CAD build for the part. Positions are in the model's coordinates, mm. A direction names the side the tool comes from. Round coordinates to 2 decimals unless told otherwise and drop trailing zeros. Loops run counter-clockwise (first coordinate to the right, second up) from the corner with the lowest first, then second, coordinate; pieces in that order, holes last.
Autodesk Inventor part; units mm, degrees
ref_plane "YZ Plane" through (0, 0, 0) normal (1, 0, 0) x (0, 1, 0)
ref_plane "XZ Plane" through (0, 0, 0) normal (0, 1, 0) x (-1, 0, 0)
ref_plane "XY Plane" through (0, 0, 0) normal (0, 0, 1) x (1, 0, 0)
sketch "Sketch1" plane through (0, 0, 0) normal (0, 0, 1) x (1, 0, 0)
  line L0 (-300, 0) -> (300, 0)
  line L1 (300, 0) -> (300, 1900)
  line L2 (300, 1900) -> (-300, 1900)
  line L3 (-300, 1900) -> (-300, 0)
  point P0 (0, 0)
  point P1 (0, 0)
  dimension "d0" = 600
  dimension "d1" = 1900
extrude "Extrusion1" add sketch "Sketch1" along normal blind 330
sketch "Sketch2" plane through (-300, 1900, 0) normal (0, 1, 0) x (1, 0, 0)
  line L0 (600, 0) -> (0, 0) construction
  line L1 (0, 0) -> (0, -330) construction
  line L2 (600, -330) -> (0, -330) construction
  line L3 (600, 0) -> (600, -330) construction
  line L4 (0, 0) -> (600, 0)
  line L5 (600, 0) -> (600, -350)
  line L6 (600, -350) -> (0, -350)
  line L7 (0, -350) -> (0, 0)
  point P0 (300, 0)
  dimension "d4" = 350
extrude "Extrusion2" add sketch "Sketch2" against normal blind 17.5
sketch "Sketch3" plane through (0, 0, 330) normal (0, 0, 1) x (1, 0, 0)
  line L0 (300, 1882.5) -> (-300, 1882.5)
  line L1 (-282.5, 1882.5) -> (282.5, 1882.5)
  line L2 (282.5, 1882.5) -> (282.5, 1575)
  line L3 (282.5, 1575) -> (-282.5, 1575)
  line L4 (-282.5, 1575) -> (-282.5, 1882.5)
  line L5 (-282.5, 1557.5) -> (282.5, 1557.5)
  line L6 (282.5, 1557.5) -> (282.5, 1250)
  line L7 (282.5, 1250) -> (-282.5, 1250)
  line L8 (-282.5, 1250) -> (-282.5, 1557.5)
  line L9 (282.5, 1232.5) -> (-282.5, 1232.5)
  line L10 (-282.5, 1232.5) -> (-282.5, 925)
  line L11 (-282.5, 925) -> (282.5, 925)
  line L12 (282.5, 925) -> (282.5, 1232.5)
  line L13 (-282.5, 907.5) -> (282.5, 907.5)
  line L14 (282.5, 907.5) -> (282.5, 600)
  line L15 (282.5, 600) -> (-282.5, 600)
  line L16 (-282.5, 600) -> (-282.5, 907.5)
  line L17 (-300, 0) -> (300, 0)
  line L18 (-282.5, 1575) -> (-282.5, 1557.5) construction
  line L19 (-282.5, 1250) -> (-282.5, 1232.5) construction
  line L20 (-282.5, 925) -> (-282.5, 907.5) construction
  point P0 (0, 0)
  point P1 (0, 600)
  point P2 (0, 0)
  dimension "d7" = 600
  dimension "d8" = 17.5
  dimension "d9" = 565
extrude "Extrusion3" cut sketch "Sketch3" against normal blind 312.5
properties part number "Libreria"
Item 1: Cut at A-A (x = 215). List the corners of the cut face in (y, z).
Verdict:
outline: (0, 0) - (1900, 0) - (1900, 350) - (1882.5, 350) - (1882.5, 17.5) - (1575, 17.5) - (1575, 330) - (1557.5, 330) - (1557.5, 17.5) - (1250, 17.5) - (1250, 330) - (1232.5, 330) - (1232.5, 17.5) - (925, 17.5) - (925, 330) - (907.5, 330) - (907.5, 17.5) - (600, 17.5) - (600, 330) - (0, 330) - close
Item 2: Wall check: L1, parallel to Y at x = -109.5, z = 62; L2, parallel to X at y = 1537, z = 296; L3, parallel to Z at x = 119.5, y = 1689. Give the ranges that are in metal, low to high.
Verdict:
L1: y = 0 to 600, 907.5 to 925, 1232.5 to 1250, 1557.5 to 1575, 1882.5 to 1900
L2: x = -300 to -282.5, 282.5 to 300
L3: z = 0 to 17.5
Item 3: Cut at C-C (y = 1175.5). List the corners of the cut face in (x, z).
Verdict:
outline: (-300, 0) - (300, 0) - (300, 330) - (282.5, 330) - (282.5, 17.5) - (-282.5, 17.5) - (-282.5, 330) - (-300, 330) - close
Item 4: Cut at D-D (y = 530). List the corners of the cut face in (x, z), plus the area to 3 significant figures.
Verdict:
outline: (-300, 0) - (300, 0) - (300, 330) - (-300, 330) - close
area: 198,000 mm2
Item 5: Flat gauge pin, fed straight in: P1, Ø3, axis at x = 230.5, y = 1240.5, coming from the +Z side. Where does the tip first touch, or does it go through?
Verdict:
P1: stops at z = 330
Item 6: Cut at B-B (z = 230). List the corners of the cut face in (x, y).
Verdict:
outline: (-300, 0) - (300, 0) - (300, 1900) - (-300, 1900) - close; hole (-282.5, 600) - (282.5, 600) - (282.5, 907.5) - (-282.5, 907.5) - close; hole (-282.5, 925) - (282.5, 925) - (282.5, 1232.5) - (-282.5, 1232.5) - close; hole (-282.5, 1250) - (282.5, 1250) - (282.5, 1557.5) - (-282.5, 1557.5) - close; hole (-282.5, 1575) - (282.5, 1575) - (282.5, 1882.5) - (-282.5, 1882.5) - close
Item 7: 3-axis set-ups, long thin cutter, end or side, ignore diameter. For faces 5 (the flat face through (-300, 963, 173)), 6 (the flat face through (-282.5, 1402, 176)): which of +Z, -Z, +X, -X, +Y, -Y reach the whole face in a straight line?
Verdict:
face 5: +Z, -Z, -X, +Y, -Y
face 6: +Z
Item 8: Mould opens along Y. For faces 1 (the flat face through (4, 1575, 176)), 2 (the flat face through (-1, 458, 330)), 3 (the flat face through (-4, 0, 163)), 4 (the flat face through (4, 1900, 173)) say: released by +Y, released by -Y, zero draft, split by the parting line, or undercut.
Verdict:
face 1: undercut
face 2: zero draft
face 3: released by -Y
face 4: released by +Y
